Autodesk Inventor part; units mm, degrees
ref_plane "YZ Plane" through (0, 0, 0) normal (1, 0, 0) x (0, 1, 0)
ref_plane "XZ Plane" through (0, 0, 0) normal (0, 1, 0) x (-1, 0, 0)
ref_plane "XY Plane" through (0, 0, 0) normal (0, 0, 1) x (1, 0, 0)
ref_plane "РабПлоскость1" through (0, 0, 0) normal (0, 0, 1) x (1, 0, 0)
sketch "Эскиз1" plane through (0, 0, 0) normal (0, 0, 1) x (1, 0, 0)
  circle A0 centre (43.2836, -60.3339) radius 1.5
  circle A1 centre (43.2836, -130.3339) radius 1.5
  circle A2 centre (43.2836, -60.3339) radius 1.6
  circle A3 centre (43.2836, -130.3339) radius 1.6
  line L0 (43.2836, -60.3339) -> (43.2836, -130.3339)
  line L1 (43.2836, -95.3339) -> (58.2836, -95.3339)
  circle A4 centre (58.2836, -95.3339) radius 2
  circle A5 centre (58.2836, -95.3339) radius 4
  line L2 (58.2836, -95.3339) -> (43.2836, -60.3339) construction
  line L3 (60.5815, -94.3491) -> (45.5815, -59.3491)
  line L4 (40.9858, -61.3187) -> (55.9858, -96.3187)
  arc A6 (55.9858, -96.3187) -> (60.5815, -94.3491) centre (58.2836, -95.3339) ccw
  arc A7 (45.5815, -59.3491) -> (40.9858, -61.3187) centre (43.2836, -60.3339) ccw
  line L5 (58.2836, -95.3339) -> (43.2836, -130.3339) construction
  line L6 (55.9858, -94.3491) -> (40.9858, -129.3491)
  line L7 (45.5815, -131.3187) -> (60.5815, -96.3187)
  arc A8 (60.5815, -96.3187) -> (55.9858, -94.3491) centre (58.2836, -95.3339) ccw
  arc A9 (40.9858, -129.3491) -> (45.5815, -131.3187) centre (43.2836, -130.3339) ccw
  point P0 (0, 0)
  point P1 (50.7836, -77.8339)
  point P2 (50.7836, -112.8339)
  point P3 (59.3515, -99.1887)
  point P4 (59.3515, -91.4791)
  point P5 (54.7558, -93.4487)
  point P6 (54.7558, -97.2191)
  dimension "d0" = 3.2
  dimension "d1" = 3.2
  dimension "d2" = 15
  dimension "d3" = 4
  dimension "d4" = 8
  dimension "d5" = 5
  dimension "d6" = 5
extrude "Выдавливание1" add sketch "Эскиз1" along normal blind 7 contours L4 A7 L3 A5 | L4 L1 A5 | A5 L3 A8 L6 L4 | L6 A5 L7 A9 | L1 L6 A5 | A5 L7 A6 L3 | L6 A8 A6 L4 | L4 A6 L7 A5 L6
properties part number "Шаблон"
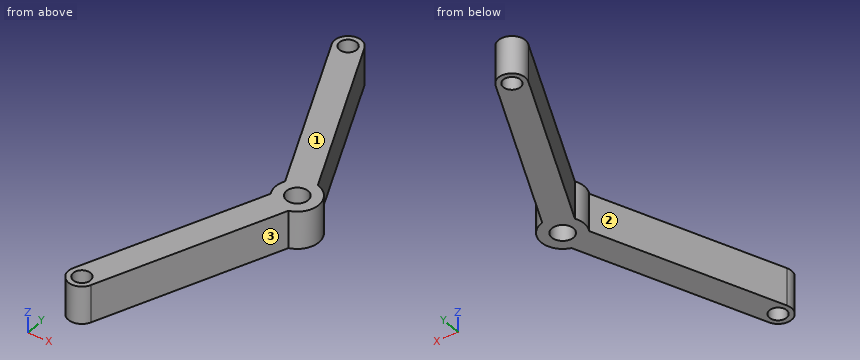
For this review, take the finished solid that the model builds, in its own axes (mm). Face numbers are marked on the shaded views. Coordinates: 2 decimals unless noted, no trailing zeros. Order: outer loops, then holes, each group sorted by start corner. A loop starts at its lowest first (then second) coordinate and runs counter-clockwise, first axis right, second up. Notation, with made-up numbers: (-4, 49.5) - (38, 49.5) arc R18 cw to (38, 67.5) - close; hole circle Ø8 at (55, 40.5). An arc over 180 degrees is marked (long way). Use one line per item in the form item = value.
Q1. Consider section A-A (x = 46.5). Give the boundary of the cut face in (y, z).
Checked values:
outline = (-129.18, 0) - (-116.48, 0) - (-116.48, 7) - (-129.18, 7) - close; (-74.19, 0) - (-61.49, 0) - (-61.49, 7) - (-74.19, 7) - close
Q2. Consider section C-C (y = -102.5). Give the boundary of the cut face in (x, z), then the cut area to 3 significant figures.
Checked values:
outline = (52.49, 0) - (57.93, 0) - (57.93, 7) - (52.49, 7) - close
area = 38.1 mm2
Q3. Consider section B-B (z = 5). Give the boundary of the cut face in (x, y).
Checked values:
outline = (40.99, -129.35) arc R2.5 ccw to (45.58, -131.32) - (59.35, -99.19) arc R4 ccw to (59.35, -91.48) - (45.58, -59.35) arc R2.5 ccw to (40.99, -61.32) - (54.76, -93.45) arc R4 ccw to (54.76, -97.22) - close; hole circle Ø3.2 at (43.28, -130.33); hole circle Ø3.2 at (43.28, -60.33); hole circle Ø4 at (58.28, -95.33)
Q4. For probe 1 along Y at (x, z) = (53.5, 6.75); probe 2 along Y at (x, z) = (50.25, 5.75); probe 3 along X at (y, z) = (-101.5, 5), list the stretches that pass through material, from the lowest coordinate up. Write a range as from..to.
Checked values:
probe_1 = -112.84..-100.15, -90.52..-77.83
probe_2 = -120.43..-107.73, -82.94..-70.24
probe_3 = 52.92..58.36
Q5. Draft analysis for pull direction Y (two halves, no side actions). For the marked faces 1, 2 and 3, state which applies: +Y half, -Y half, draft (parallel to the pull), parting line (faces both ways), or undercut.
Checked values:
face_1 = draft
face_2 = undercut
face_3 = -Y half
Q6. For P1, Ø3, axis at x = 56, z = 1, coming from the +Y side; P2, Ø6, axis at x = 44.5, y = -78, coming from the +Z side; P3, Ø4, axis at x = 47, z = 2.5, coming from the +Y side; P4, Ø2, axis at x = 53, z = 3.5, coming from the +Y side, all flat-tipped, find the tip position at first contact; note any pin that passes through.
Checked values:
P1 = -80.16
P2 = through
P3 = -58.52
P4 = -74.33
